```python
from build123d import *

# Parameters (mm, degrees)
SKETCH1_W           = 120
SKETCH1_H           = 171.827864376
SKETCH1_R           = 1.5
SKETCH1_W_2         = 114
SKETCH1_H_2         = 37
BOSS_EXTRUDE1_DEPTH = 4
SKETCH2_W           = 9
SKETCH2_H           = 14.6
CUT_EXTRUDE1_DEPTH  = 5


with BuildPart() as part:
    # Sketch1 → Boss-Extrude1 (new body)
    with BuildSketch(Plane.XY):
        with Locations((60, 77.985)):
            Rectangle(SKETCH1_W, SKETCH1_H)
        with Locations((13, 150.313145751)):
            Circle(SKETCH1_R, mode=Mode.SUBTRACT)
        with Locations((107, 150.313145751)):
            Circle(SKETCH1_R, mode=Mode.SUBTRACT)
        with Locations((109.5, 0.156854249)):
            Circle(SKETCH1_R, mode=Mode.SUBTRACT)
        with Locations((12, 0)):
            Circle(SKETCH1_R, mode=Mode.SUBTRACT)
        with Locations((60, 122.47)):
            Rectangle(SKETCH1_W_2, SKETCH1_H_2, mode=Mode.SUBTRACT)
        Polygon((31.5, 143.97), (27.5, 143.97), (27.5, 145.97), (35.5, 145.97), (35.5, 143.97), align=None, mode=Mode.SUBTRACT)
        Polygon((92.5, 145.97), (84.5, 145.97), (84.5, 143.97), (88.5, 143.97), (92.5, 143.97), align=None, mode=Mode.SUBTRACT)
        Polygon((60, 98.97), (56, 98.97), (56, 100.97), (64, 100.97), (64, 98.97), align=None, mode=Mode.SUBTRACT)
    extrude(amount=BOSS_EXTRUDE1_DEPTH)

    # Sketch2 → Cut-Extrude1 (cut, through all)
    with BuildSketch(Plane(origin=(0, 0, 0), x_dir=(-1, 0, 0), z_dir=(0, 0, -1))):
        with Locations((-78.856585714, 64.426127197)):
            Rectangle(SKETCH2_W, SKETCH2_H)
    extrude(amount=-CUT_EXTRUDE1_DEPTH, mode=Mode.SUBTRACT)


solid = part.part
```
Input: part model. Units: mm. Frame: model coordinates. A direction names the side the tool comes from. Round coordinates to 2 decimals unless told otherwise and drop trailing zeros. Order: outer loops, then holes, each group sorted by start corner. A loop starts at its lowest first (then second) coordinate and runs counter-clockwise, first axis right, second up. Notation, with made-up numbers: (54.25, 30) - (78.25, 30) arc R19 cw to (78.25, 39) - close; hole circle Ø10 at (26, -29). An arc over 180 degrees is marked (long way). Answer in a Markdown table with one row per item.
Item 1: Section query A-A (y = 135). Return the cut outline in (x, z).
Model answer:
| item | result |
|---|---|
| outline | (0, 0) - (3, 0) - (3, 4) - (0, 4) - close; (117, 0) - (120, 0) - (120, 4) - (117, 4) - close |
Item 2: Section query B-B (x = 100.5). Return the cut outline in (y, z).
Model answer:
| item | result |
|---|---|
| outline | (-7.93, 0) - (103.97, 0) - (103.97, 4) - (-7.93, 4) - close; (140.97, 0) - (163.9, 0) - (163.9, 4) - (140.97, 4) - close |
Item 3: Reachability of faces 1 (the flat face through (59, -7.929, 2)), 2 (the flat face through (117, 122, 2)) from +Z, -Z, +X, -X, +Y, -Y: full face, straight path, thin tool, end or side. Return the list, or none.
Model answer:
| item | result |
|---|---|
| face 1 | +Z, -Z, +X, -X, -Y |
| face 2 | +Z, -Z |
Item 4: Mould query, pull axis X, two halves, no side actions, for faces 3 (the flat face through (59, 60, 0)), 4 (the flat face through (0, 77, 2)), 5 (the flat face through (89, 143.97, 2)). Classes: released by +X, released by -X, zero draft, split by the parting line, or undercut.
Model answer:
| item | result |
|---|---|
| face 3 | zero draft |
| face 4 | released by -X |
| face 5 | undercut |
Item 5: Line query: line 1 (Y direction, x = 34, z = 2.85); line 2 (Y direction, x = 107, z = 1.4); line 3 (X direction, y = 150.5, z = 1.9). Output: solid intervals per line, ascending.
Model answer:
| item | result |
|---|---|
| line 1 | y = -7.93 to 103.97, 140.97 to 143.97, 145.97 to 163.9 |
| line 2 | y = -7.93 to 103.97, 140.97 to 148.81, 151.81 to 163.9 |
| line 3 | x = 0 to 11.51, 14.49 to 105.51, 108.49 to 120 |
Item 6: Section query C-C (z = 1.15). Give the number of separate pieces and of enclosed holes in the cut face, then the cut area to 3 significant figures.
Model answer:
| item | result |
|---|---|
| separate pieces | 1 |
| enclosed holes | 9 |
| area | 16,200 mm² |
Item 7: Pin query (flat end, axial travel): pin 1 (1.8 mm diameter, centred on x = 12, y = 0, fed in from +Z); pin 2 (1.6 mm diameter, centred on y = 145, z = 1, fed in from -X). Return the tip coordinate at first contact, or that it passes through.
Model answer:
| item | result |
|---|---|
| pin 1 | passes through |
| pin 2 | stops at x = 0 |
